Part model, mm, in its own coordinate system. Face numbers are marked on the shaded views. A direction names the side the tool comes from. Coordinates: 2 decimals unless noted, no trailing zeros. Loops run counter-clockwise (first coordinate to the right, second up) from the corner with the lowest first, then second, coordinate; pieces in that order, holes last. Notation, with made-up numbers: (71, 52) - (93, 52) arc R16 ccw to (93, 79) - close; hole circle Ø4 at (-31.5, -33). An arc over 180 degrees is marked (long way). Use a Markdown table: item, result. Add a question column.
1) Drop flat-ended pins along their axis: P1, Ø0.6, axis at y = -1, z = 2, coming from the -X side; P2, Ø2.5, axis at x = -15.65, z = 4, coming from the -Y side; P3, Ø2.5, axis at x = -15.5, z = 5.5, coming from the -Y side. Give the stop position or say it passes through.
2) Probe probe 1 along Z at (x, y) = (-15.65, -1.25); probe 2 along Y at (x, z) = (-11, -69); probe 3 along Y at (x, z) = (-2, -23.5). List the from-to ranges inside material, lowest first. Write a range as [from, to].
3) Band-saw the part on B-B (z = -70.5). Give the cut face in (x, y), plus the area to 3 significant figures.
4) Band-saw the part on A-A (y = -15.5). Give the cut face in (x, z).
5) Tool access for the marked faces 1, 2 and 3: list every direction of +Z, -Z, +X, -X, +Y, -Y with a clear straight run to the whole face (end or side of a thin tool).
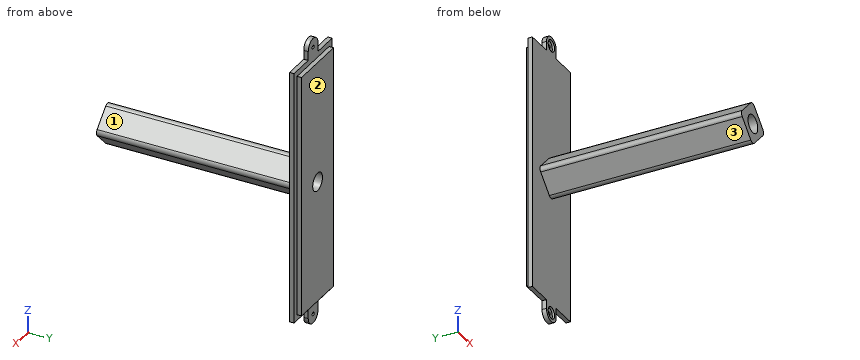
Autodesk Inventor part; units mm, degrees
ref_plane "YZ Plane" through (0, 0, 0) normal (1, 0, 0) x (0, 1, 0)
ref_plane "XZ Plane" through (0, 0, 0) normal (0, 1, 0) x (-1, 0, 0)
ref_plane "XY Plane" through (0, 0, 0) normal (0, 0, 1) x (1, 0, 0)
sketch "Esboço1" plane through (0, 0, 0) normal (0, 1, 0) x (-1, 0, 0)
  line L0 (0, 0) -> (31.3, 0)
  line L1 (31.3, 0) -> (31.3, -113.5)
  line L2 (31.3, -113.5) -> (0, -113.5)
  line L3 (0, -113.5) -> (0, 0)
  line L4 (28.8, -111) -> (28.8, -2.5)
  line L5 (28.8, -2.5) -> (2.5, -2.5)
  line L6 (2.5, -2.5) -> (2.5, -111)
  line L7 (2.5, -111) -> (28.8, -111)
  dimension "d0" = 31.3
  dimension "d1" = 113.5
  dimension "d2" = 2.5
extrude "Extrusão1" add sketch "Esboço1" along normal blind 2 contours L7 L6 L5 L4
extrude "Extrusão2" add sketch "Esboço1" against normal blind 2 contours L0 L1 L2 L3 | L7 L6 L5 L4
sketch "Esboço2" plane through (0, -2, 0) normal (0, -1, 0) x (1, 0, 0)
  line L0 (0, -113.5) -> (0, 0)
  line L1 (-15.65, 0) -> (-11.65, 0)
  line L2 (-11.65, 0) -> (-11.65, 4)
  line L3 (-19.65, 0) -> (-15.65, 0)
  line L4 (-28.8, -2.5) -> (-2.5, -2.5)
  circle A0 centre (-15.65, 4) radius 0.8
  line L5 (0, 0) -> (0, -113.5)
  line L6 (-19.65, 0) -> (-19.65, 4)
  arc A1 (-11.65, 4) -> (-19.65, 4) centre (-15.65, 4) ccw
  line L7 (-31.3, -113.5) -> (-31.3, 0)
  line L8 (-15.65, -113.5) -> (-11.65, -113.5)
  line L9 (-11.65, -113.5) -> (-11.65, -117.5)
  line L10 (-19.65, -113.5) -> (-15.65, -113.5)
  circle A2 centre (-15.65, -117.5) radius 0.8
  line L11 (-19.65, -113.5) -> (-19.65, -117.5)
  arc A3 (-19.65, -117.5) -> (-11.65, -117.5) centre (-15.65, -117.5) ccw
  dimension "d16" = 1.6
  dimension "d28" = 0
extrude "Extrusão3" add sketch "Esboço2" against normal blind 2
sketch "Esboço3" plane through (0, -2, 0) normal (0, -1, 0) x (1, 0, 0)
  circle A0 centre (-15.65, -56.75) radius 4
  line L0 (0, -113.5) -> (0, 0)
  line L1 (-31.3, 0) -> (-31.3, -113.5)
  line L2 (0, -113.5) -> (-31.3, -113.5)
  dimension "d18" = 8
  dimension "d21" = 15.65
  dimension "d33" = 56.75
extrude "Extrusão4" cut sketch "Esboço3" against normal up to surface (4 mm away)
sketch "Esboço4" plane through (0, -2, 0) normal (0, -1, 0) x (1, 0, 0)
  circle A0 centre (-15.65, 4) radius 0.8
  circle A1 centre (-15.65, 4) radius 2.6
  line L0 (0, -113.5) -> (0, 0)
  circle A2 centre (-15.65, -117.5) radius 2.6
  dimension "d29" = 5.2
extrude "Extrusão5" cut sketch "Esboço4" against normal blind 1
sketch "Esboço5" plane through (0, -2, 0) normal (0, -1, 0) x (1, 0, 0)
  point P0 (0, 0)
sketch "Esboço6" plane through (0, -2, 0) normal (0, -1, 0) x (1, 0, 0)
  line L0 (-17.3312, -47.9978) -> (-24.4022, -55.0688)
  line L1 (-24.4022, -57.8973) -> (-17.3312, -64.9683)
  line L2 (-14.5027, -64.9683) -> (-7.4317, -57.8973)
  line L3 (-7.4317, -55.0688) -> (-14.5027, -47.9978)
  circle A0 centre (-15.65, -56.75) radius 4
  line L4 (-15.917, -46.5835) -> (-15.917, -66.3825) construction
  line L5 (-25.8165, -56.483) -> (-6.0175, -56.483) construction
  arc A1 (-24.4022, -55.0688) -> (-24.4022, -57.8973) centre (-22.988, -56.483) ccw
  arc A2 (-17.3312, -64.9683) -> (-14.5027, -64.9683) centre (-15.917, -63.5541) ccw
  arc A3 (-7.4317, -57.8973) -> (-7.4317, -55.0688) centre (-8.8459, -56.483) ccw
  arc A4 (-14.5027, -47.9978) -> (-17.3312, -47.9978) centre (-15.917, -49.412) ccw
  point P0 (0, 0)
  dimension "d34" = 14
  dimension "d35" = 2
  dimension "d38" = 14
extrude "Extrusão6" add sketch "Esboço6" along normal blind 90
properties part number "Tampa Suporte 4E_3DPrint"
Answer block:
| question | item | result |
|---|---|---|
| 1 | P1 | x = -19.65 |
| 1 | P2 | y = -1 |
| 1 | P3 | y = -2 |
| 2 | probe 1 | [-121.5, -120.1], [-114.9, -60.75], [-52.75, 1.4], [6.6, 8] |
| 2 | probe 2 | [-2, 2] |
| 2 | probe 3 | [-2, 0] |
| 3 | outline | (-31.3, -2) - (0, -2) - (0, 0) - (-2.5, 0) - (-2.5, 2) - (-28.8, 2) - (-28.8, 0) - (-31.3, 0) - close |
| 3 | area | 115 mm2 |
| 4 | outline | (-24.4, -57.9) - (-17.33, -64.97) arc R2 ccw to (-14.5, -64.97) - (-7.43, -57.9) arc R2 ccw to (-7.43, -55.07) - (-14.5, -48) arc R2 ccw to (-17.33, -48) - (-24.4, -55.07) arc R2 ccw to start; hole circle Ø8 at (-15.65, -56.75) |
| 5 | face 1 | +Z, +X, -Y |
| 5 | face 2 | +Z, -Z, +X, -X, +Y |
| 5 | face 3 | -Z, -X, -Y |
